```python
from build123d import *

# Parameters (mm, degrees)
SALIENTE_EXTRUIR1_DEPTH = 20
SALIENTE_EXTRUIR2_DEPTH = 2
SALIENTE_EXTRUIR3_DEPTH = 2
CROQUIS4_R              = 4
CORTAR_EXTRUIR1_DEPTH   = 2
CROQUIS5_R              = 4
CORTAR_EXTRUIR2_DEPTH   = 2
CORTAR_EXTRUIR3_DEPTH   = 2
CROQUIS7_R              = 1.5
CORTAR_EXTRUIR4_DEPTH   = 2
CROQUIS8_R              = 1.5
CORTAR_EXTRUIR5_DEPTH   = 2


with BuildPart() as part:
    # Croquis1 → Saliente-Extruir1 (new body)
    with BuildSketch(Plane.XY):
        Polygon((-12, 25.8), (12, 25.8), (12, -25.8), (-12, -25.8), (-14, -25.8), (-14, -27.8), (14, -27.8), (14, 27.8), (-14, 27.8), (-14, 25.8), align=None)
    extrude(amount=SALIENTE_EXTRUIR1_DEPTH)

    # Croquis2 → Saliente-Extruir2 (add)
    with BuildSketch(Plane(origin=(0, 27.8, 0), x_dir=(1, 0, 0), z_dir=(0, 1, 0))):
        with BuildLine():
            Line((-14, -20), (-14, 0))
            ThreePointArc((-14, 0), (-24, -10), (-14, -20))
        make_face()
    extrude(amount=-SALIENTE_EXTRUIR2_DEPTH)

    # Croquis3 → Saliente-Extruir3 (add)
    with BuildSketch(Plane(origin=(0, -25.8, 0), x_dir=(1, 0, 0), z_dir=(0, 1, 0))):
        with BuildLine():
            Line((-14, -20), (-14, 0))
            ThreePointArc((-14, 0), (-24, -10), (-14, -20))
        make_face()
    extrude(amount=-SALIENTE_EXTRUIR3_DEPTH)

    # Croquis4 → Cortar-Extruir1 (cut)
    with BuildSketch(Plane(origin=(0, 27.8, 0), x_dir=(1, 0, 0), z_dir=(0, 1, 0))):
        with Locations((-14, -10)):
            Circle(CROQUIS4_R)
    extrude(amount=-CORTAR_EXTRUIR1_DEPTH, mode=Mode.SUBTRACT)

    # Croquis5 → Cortar-Extruir2 (cut)
    with BuildSketch(Plane(origin=(0, -25.8, 0), x_dir=(1, 0, 0), z_dir=(0, 1, 0))):
        with Locations((-14, -10)):
            Circle(CROQUIS5_R)
    extrude(amount=-CORTAR_EXTRUIR2_DEPTH, mode=Mode.SUBTRACT)

    # Croquis6 → Cortar-Extruir3 (cut)
    with BuildSketch(Plane(origin=(14, 0, 0), x_dir=(0, 0, -1), z_dir=(1, 0, 0))):
        with BuildLine():
            ThreePointArc((-6, 0), (-7.699530032, 3.272283289), (-11.353918963, 3.763894717))
            Line((-11.353918963, 3.763894717), (-8.646081037, -3.763894717))
            ThreePointArc((-8.646081037, -3.763894717), (-6.727716711, -2.300469968), (-6, 0))
        make_face()
        with BuildLine():
            Line((-8.646081037, -3.763894717), (-11.353918963, 3.763894717))
            ThreePointArc((-11.353918963, 3.763894717), (-13.763894717, -1.353918963), (-8.646081037, -3.763894717))
        make_face()
    extrude(amount=-CORTAR_EXTRUIR3_DEPTH, mode=Mode.SUBTRACT)

    # Croquis7 → Cortar-Extruir4 (cut)
    with BuildSketch(Plane(origin=(14, 0, 0), x_dir=(0, 0, -1), z_dir=(1, 0, 0))):
        with Locations((-10, 7)):
            Circle(CROQUIS7_R)
        with Locations((-3, 0)):
            Circle(CROQUIS7_R)
        with Locations((-10, -7)):
            Circle(CROQUIS7_R)
        with Locations((-17, 0)):
            Circle(CROQUIS7_R)
    extrude(amount=-CORTAR_EXTRUIR4_DEPTH, mode=Mode.SUBTRACT)

    # Croquis8 → Cortar-Extruir5 (cut)
    with BuildSketch(Plane(origin=(14, 0, 0), x_dir=(0, 0, -1), z_dir=(1, 0, 0))):
        with Locations((-10, 18.6)):
            Circle(CROQUIS8_R)
        with Locations((-10, -18.6)):
            Circle(CROQUIS8_R)
    extrude(amount=-CORTAR_EXTRUIR5_DEPTH, mode=Mode.SUBTRACT)


solid = part.part
```
Geometry check sheet. Reference: the model listing, model coordinates, mm. A direction names the side the tool comes from. Give positions to 0.01 mm unless a question says otherwise; leave off trailing zeros. Write each loop counter-clockwise with the first axis right and the second up, starting at its lowest first coordinate (ties: lowest second). Pieces come first, ordered by that corner, then holes. Notation, with made-up numbers: (-3.5, -9) -> (12.5, -9) arc R36 ccw to (12.5, 29) -> close; hole circle Ø8 at (8.5, 45). An arc over 180 degrees is marked (long way). Use one line per item in the form item = value.
Item 1: Sectioned sample at A-A on x = -4.5. Enter the section's corners in (y, z).
Results list:
outline = (-27.8, 0) -> (-25.8, 0) -> (-25.8, 20) -> (-27.8, 20) -> close; (25.8, 0) -> (27.8, 0) -> (27.8, 20) -> (25.8, 20) -> close
Item 2: Sectioned sample at D-D on z = 7. Enter the section's corners in (x, y), plus the area to 3 significant figures.
Results list:
outline = (-23.54, -27.8) -> (-16.65, -27.8) -> (-16.65, -25.8) -> (-23.54, -25.8) -> close; (-23.54, 25.8) -> (-16.65, 25.8) -> (-16.65, 27.8) -> (-23.54, 27.8) -> close; (-11.35, -27.8) -> (14, -27.8) -> (14, -2.65) -> (12, -2.65) -> (12, -25.8) -> (-11.35, -25.8) -> close; (-11.35, 25.8) -> (12, 25.8) -> (12, 2.65) -> (14, 2.65) -> (14, 27.8) -> (-11.35, 27.8) -> close
area = 222 mm2
Item 3: Scan lines: line 1 (Y direction, x = 13.1, z = 10); line 2 (Y direction, x = 10, z = 11.5); line 3 (Z direction, x = -14, y = 26.9). Record each from-to range of solid material in increasing order.
Results list:
line_1 = -27.8 to -20.1, -17.1 to -8.5, -5.5 to -4, 4 to 5.5, 8.5 to 17.1, 20.1 to 27.8
line_2 = -27.8 to -25.8, 25.8 to 27.8
line_3 = 0 to 6, 14 to 20
Item 4: Mould release check, pull along Z, two halves, no side actions. Record for faces 3 (the cylindrical face through (13.01, 0.45, 1.57)), 4 (the flat face through (12.4, 0.1, 20)), 5 (the cylindrical face through (13, 6.1, 11.2)), 6 (the flat face through (-5, -27.8, 10)): released by +Z, released by -Z, zero draft, split by the parting line, or undercut.
Results list:
face_3 = undercut
face_4 = released by +Z
face_5 = undercut
face_6 = zero draft
Item 5: Depth check by flat-ended pin: pin 1 Ø10 at (y, z) = (-2.5, 14.5) entering from -X. Enter the tip coordinate at first touch or a pass-through.
Results list:
pin_1 = 12
Item 6: Sectioned sample at B-B on y = 18.6. Enter the section's corners in (x, z), plus the area to 3 significant figures.
Results list:
outline = (12, 0) -> (14, 0) -> (14, 8.5) -> (12, 8.5) -> close; (12, 11.5) -> (14, 11.5) -> (14, 20) -> (12, 20) -> close
area = 34.0 mm2
Item 7: Access from +Z, -Z, +X, -X, +Y, -Y to the whole of each face (thin tool, end or side, straight path). Record for faces 1 (the flat face through (-6, 25.8, 10)), 2 (the cylindrical face through (13, -7.9, 11.2)).
Results list:
face_1 = +Z, -Z, -X
face_2 = +X, -X
Item 8: Sectioned sample at C-C on z = 17. Enter the section's corners in (x, y).
Results list:
outline = (-21.14, -27.8) -> (14, -27.8) -> (14, -1.5) -> (12, -1.5) -> (12, -25.8) -> (-21.14, -25.8) -> close; (-21.14, 25.8) -> (12, 25.8) -> (12, 1.5) -> (14, 1.5) -> (14, 27.8) -> (-21.14, 27.8) -> close
